Input: part model. Units: mm. Frame: model coordinates. Coordinates: 2 decimals unless noted, no trailing zeros. Order: outer loops, then holes, each group sorted by start corner. A loop starts at its lowest first (then second) coordinate and runs counter-clockwise, first axis right, second up. Notation, with made-up numbers: M 61.25,17 L 94.25,17 A20 cw 94.25,35 Z; hole C 81.5,17 d3. An arc over 180 degrees is marked long. Answer in a Markdown table with one row per item.
from build123d import *

# Parameters (mm, degrees)
SKETCH1_W           = 18
SKETCH1_H           = 20
SKETCH1_R           = 1
BOSS_EXTRUDE1_DEPTH = 1
SKETCH2_R           = 0.75
CUT_EXTRUDE1_DEPTH  = 1
SKETCH3_W           = 10.1
SKETCH3_H           = 3.86
BOSS_EXTRUDE3_DEPTH = 0.5
SKETCH4_W           = 0.9
SKETCH4_H           = 1.9
SKETCH4_W_2         = 1.65
SKETCH4_H_2         = 3.65
BOSS_EXTRUDE4_DEPTH = 0.5


with BuildPart() as part:
    # Sketch1 → Boss-Extrude1 (new body)
    with BuildSketch(Plane.XY):
        Rectangle(SKETCH1_W, SKETCH1_H)
        with Locations((7.65, 8.5)):
            Circle(SKETCH1_R, mode=Mode.SUBTRACT)
        with Locations(Location((7.65, -8.5, 0), (0, 0, 180))):
            Circle(SKETCH1_R, mode=Mode.SUBTRACT)
    extrude(amount=BOSS_EXTRUDE1_DEPTH)

    # Sketch2 → Cut-Extrude1 (cut)
    with BuildSketch(Plane.XY.offset(1)):
        with Locations((-7.53, 6.9)):
            Circle(SKETCH2_R)
        with Locations((-7.53, 4.36)):
            Circle(SKETCH2_R)
        with Locations((-7.53, 1.82)):
            Circle(SKETCH2_R)
        with Locations((-7.53, -0.72)):
            Circle(SKETCH2_R)
        with Locations((-7.53, -3.26)):
            Circle(SKETCH2_R)
        with Locations((-7.53, -5.8)):
            Circle(SKETCH2_R)
        with Locations(Location((7.53, -3.26, 0), (0, 0, 180))):
            Circle(SKETCH2_R)
        with Locations(Location((7.53, -0.72, 0), (0, 0, 180))):
            Circle(SKETCH2_R)
        with Locations(Location((7.53, 1.82, 0), (0, 0, 180))):
            Circle(SKETCH2_R)
        with Locations(Location((7.53, 4.36, 0), (0, 0, 180))):
            Circle(SKETCH2_R)
    extrude(amount=-CUT_EXTRUDE1_DEPTH, mode=Mode.SUBTRACT)

    # Sketch3 → Boss-Extrude3 (add)
    with BuildSketch(Plane.XY.offset(1)):
        Rectangle(SKETCH3_W, SKETCH3_H)
    extrude(amount=BOSS_EXTRUDE3_DEPTH)

    # Sketch4 → Boss-Extrude4 (add)
    with BuildSketch(Plane.XY.offset(1)):
        with Locations((-4.519825255, 6.542108994)):
            Rectangle(SKETCH4_W, SKETCH4_H)
        with Locations((-3.070068301, 6.542108994)):
            Rectangle(SKETCH4_W, SKETCH4_H)
        with Locations((-1.482219023, 6.522505917)):
            Rectangle(SKETCH4_W, SKETCH4_H)
        with Locations((0.105630256, 6.502902839)):
            Rectangle(SKETCH4_W, SKETCH4_H)
        with Locations((1.782648632, 6.524274443)):
            Rectangle(SKETCH4_W, SKETCH4_H)
        with Locations((3.910298039, 7.361938069)):
            Rectangle(SKETCH4_W_2, SKETCH4_H_2)
        with Locations((3.910298039, -7.361938069)):
            Rectangle(SKETCH4_W_2, SKETCH4_H_2)
        with Locations((1.782648632, -6.524274443)):
            Rectangle(SKETCH4_W, SKETCH4_H)
        with Locations((0.105630256, -6.502902839)):
            Rectangle(SKETCH4_W, SKETCH4_H)
        with Locations((-1.482219023, -6.522505917)):
            Rectangle(SKETCH4_W, SKETCH4_H)
        with Locations((-3.070068301, -6.542108994)):
            Rectangle(SKETCH4_W, SKETCH4_H)
        with Locations((-4.519825255, -6.542108994)):
            Rectangle(SKETCH4_W, SKETCH4_H)
    extrude(amount=BOSS_EXTRUDE4_DEPTH)


solid = part.part
1) Mould query, pull axis Y, two halves, no side actions, for faces 1 (the face through (-6.84, -3.55, 0.51)), 2 (the face through (-0.1, -10, 0.5)), 3 (the face through (-0.1, 10, 0.5)), 4 (the face through (-9, -0.1, 0.5)). Classes: +Y half, -Y half, draft (parallel to the pull), parting line (faces both ways), or undercut.
Resolved:
| item | result |
|---|---|
| face 1 | undercut |
| face 2 | -Y half |
| face 3 | +Y half |
| face 4 | draft |
2) Cut plane D-D, the plane x = -7.53. Output: boundary loops of the cut face in (y, z), and give its area (3 significant figures).
Resolved:
| item | result |
|---|---|
| outline | M -10,0 L -6.55,0 L -6.55,1 L -10,1 Z; M -5.05,0 L -4.01,0 L -4.01,1 L -5.05,1 Z; M -2.51,0 L -1.47,0 L -1.47,1 L -2.51,1 Z; M 0.03,0 L 1.07,0 L 1.07,1 L 0.03,1 Z; M 2.57,0 L 3.61,0 L 3.61,1 L 2.57,1 Z; M 5.11,0 L 6.15,0 L 6.15,1 L 5.11,1 Z; M 7.65,0 L 10,0 L 10,1 L 7.65,1 Z |
| area | 11.0 mm2 |
3) Cut plane C-C, the plane z = 0.7. State how many separate pieces and enclosed holes the cut face has, and give its area (3 significant figures).
Resolved:
| item | result |
|---|---|
| separate pieces | 1 |
| enclosed holes | 12 |
| area | 336 mm2 |
4) Cut plane B-B, the plane y = -8.5. Output: boundary loops of the cut face in (x, z).
Resolved:
| item | result |
|---|---|
| outline | M -9,0 L 6.65,0 L 6.65,1 L 4.74,1 L 4.74,1.5 L 3.09,1.5 L 3.09,1 L -9,1 Z; M 8.65,0 L 9,0 L 9,1 L 8.65,1 Z |
5) Cut plane A-A, the plane y = -3.26. Output: boundary loops of the cut face in (x, z), and give its area (3 significant figures).
Resolved:
| item | result |
|---|---|
| outline | M -9,0 L -8.28,0 L -8.28,1 L -9,1 Z; M -6.78,0 L 6.78,0 L 6.78,1 L -6.78,1 Z; M 8.28,0 L 9,0 L 9,1 L 8.28,1 Z |
| area | 15.0 mm2 |
6) Contact query for flat-ended pins moving along their axis: pin 1 (3 mm diameter, centred on x = 1.5, y = -6, fed in from -Z); pin 2 (1.5 mm diameter, centred on x = -6, y = -6, fed in from +Z); pin 3 (0.6 mm diameter, centred on y = 6.5, z = 1.5, fed in from -X); pin 4 (1.8 mm diameter, centred on x = 7.65, y = -8.5, fed in from +Z). Output: stop coordinate, or through.
Resolved:
| item | result |
|---|---|
| pin 1 | stops at z = 0 |
| pin 2 | stops at z = 1 |
| pin 3 | stops at x = -4.97 |
| pin 4 | passes through |
7) Material intervals for probe 1 along X at (y, z) = (6.25, 1.35); probe 2 along X at (y, z) = (-3.5, 0.7); probe 3 along X at (y, z) = (-1.25, 0.4), sorted ascending.
Resolved:
| item | result |
|---|---|
| probe 1 | x = -4.97 to -4.07, -3.52 to -2.62, -1.93 to -1.03, -0.34 to 0.56, 1.33 to 2.23, 3.09 to 4.74 |
| probe 2 | x = -9 to -8.24, -6.82 to 6.82, 8.24 to 9 |
| probe 3 | x = -9 to -8.06, -7 to 7, 8.06 to 9 |
